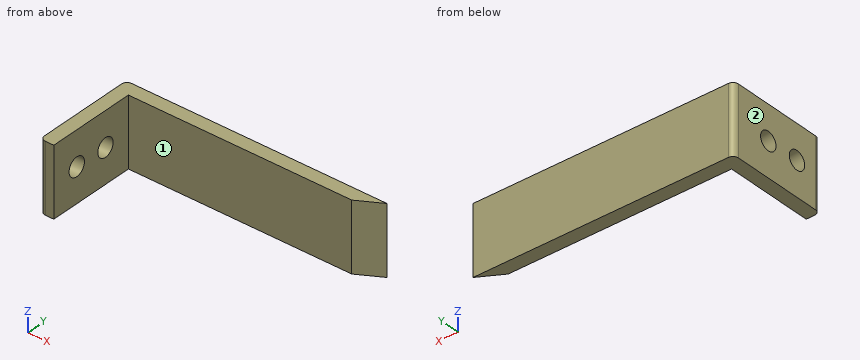
Autodesk Inventor part; units mm, degrees
ref_plane "YZ Plane" through (0, 0, 0) normal (1, 0, 0) x (0, 1, 0)
ref_plane "XZ Plane" through (0, 0, 0) normal (0, 1, 0) x (-1, 0, 0)
ref_plane "XY Plane" through (0, 0, 0) normal (0, 0, 1) x (1, 0, 0)
sketch "Sketch1" plane through (0, 0, 0) normal (0, 1, 0) x (-1, 0, 0)
  line L0 (0, 6.35) -> (-45.72, 6.35)
  line L1 (-45.72, 6.35) -> (-45.72, -6.35)
  line L2 (-45.72, -6.35) -> (0, -6.35)
  line L3 (0, -6.35) -> (0, 6.35)
  point P0 (0, 0)
  dimension "d0" = 45.72
  dimension "d1" = 12.7
  dimension "d2" = 6.35
extrude "Extrusion1" add sketch "Sketch1" along normal blind 2.54
sketch "Sketch2" plane through (0, 2.54, 0) normal (0, 1, 0) x (1, 0, 0)
  line L0 (0, 6.35) -> (0, -6.35)
  line L1 (0, 6.35) -> (-2.54, 6.35)
  line L2 (-2.54, 6.35) -> (-2.54, -6.35)
  line L3 (-2.54, -6.35) -> (0, -6.35)
  line L4 (0, -6.35) -> (0, 6.35)
  point P0 (0, 0)
  point P1 (0, -6.35)
  dimension "d5" = 2.54
extrude "Extrusion2" add sketch "Sketch2" against normal blind 19.05
sketch "Sketch3" plane through (0, -16.51, 6.35) normal (1, 0, 0) x (0, 0, -1)
  circle A0 centre (6.35, 11.43) radius 1.7
  circle A1 centre (6.35, 5.08) radius 1.7
  line L0 (12.7, 16.51) -> (0, 16.51)
  point P0 (6.35, 16.51)
  dimension "d8" = 3.4
  dimension "d9" = 3.4
  dimension "d10" = 5.08
  dimension "d11" = 6.35
extrude "Extrusion3" cut sketch "Sketch3" against normal through all
fillet "Fillet1" radius 1.016 2 edges at (-2.54, 2.54, 0) (-2.54, -16.51, 0)
sketch "Sketch4" plane through (45.72, 0, 6.35) normal (0, 0, 1) x (1, 0, 0)
  line L0 (0, 0) -> (0, 2.54)
  line L1 (0, 2.54) -> (-4.3994, 0)
  line L2 (-45.72, 0) -> (0, 0)
  line L3 (0, 2.54) -> (5.08, 2.54) construction
  line L4 (-4.3994, 0) -> (0, 0)
  line L5 (0, 0) -> (0, 2.54)
  dimension "d15" = 150
extrude "Extrusion4" cut sketch "Sketch4" against normal through all
properties part number "capstone ear"
CAD build for the part. Positions are in the model's coordinates, mm. Face numbers are marked on the shaded views. A direction names the side the tool comes from. Coordinates: 2 decimals unless noted, no trailing zeros. Write each loop counter-clockwise with the first axis right and the second up, starting at its lowest first coordinate (ties: lowest second). Pieces come first, ordered by that corner, then holes. Notation, with made-up numbers: M -5,26 L 4,26 A23 ccw 4,51 Z; hole C 7,4.5 d5. An arc over 180 degrees is marked long. Answer as a JSON object with one key per item and string values. Group by question number.
1) Tool access for the marked faces 1 and 2: list every direction of +Z, -Z, +X, -X, +Y, -Y with a clear straight run to the whole face (end or side of a thin tool).
2) Saw through at A-A (y = -11.43). Write the cut outline in (x, z), plus the area to 3 significant figures.
3) Wall check: line 1 (Y direction, x = -1.35, z = 0); line 2 (X direction, y = -2.75, z = -1.25); line 3 (Y direction, x = 25, z = -4.25). Give the ranges that are in metal, low to high. Write a range as from..to.
4) Pin check, flat tip, straight feed: pin 1 Ø4 at (x, z) = (14.5, 3.5) entering from -Y. Stop position of the tip, or through.
5) Saw through at B-B (z = 0). Write the cut outline in (x, y), plus the area to 3 significant figures.
6) Saw through at D-D (x = 30). Write the cut outline in (y, z).
7) Saw through at C-C (z = 4.25). Write the cut outline in (x, y), plus the area to 3 significant figures.
Values follow:
{
 "1": {"face 1": "+Z, -Z, +X, -Y", "face 2": "+Z, -Z, -X, +Y, -Y"},
 "2": {"outline": "M -2.54,-6.35 L 0,-6.35 L 0,-1.7 L -2.54,-1.7 Z; M -2.54,1.7 L 0,1.7 L 0,6.35 L -2.54,6.35 Z", "area": "23.6 mm2"},
 "3": {"line 1": "y = -16.51..-13.13, -9.73..-6.78, -3.38..2.54", "line 2": "x = -2.54..0", "line 3": "y = 0..2.54"},
 "4": {"pin 1": "stops at y = 0"},
 "5": {"outline": "M -2.54,-15.49 A1.02 ccw -1.52,-16.51 L 0,-16.51 L 0,-13.13 L -2.54,-13.13 Z; M -2.54,-9.73 L 0,-9.73 L 0,-6.78 L -2.54,-6.78 Z; M -2.54,-3.38 L 0,-3.38 L 0,0 L 41.32,0 L 45.72,2.54 L -1.52,2.54 A1.02 ccw -2.54,1.52 Z", "area": "141 mm2"},
 "6": {"outline": "M 0,-6.35 L 2.54,-6.35 L 2.54,6.35 L 0,6.35 Z"},
 "7": {"outline": "M -2.54,-15.49 A1.02 ccw -1.52,-16.51 L 0,-16.51 L 0,0 L 41.32,0 L 45.72,2.54 L -1.52,2.54 A1.02 ccw -2.54,1.52 Z", "area": "158 mm2"}
}
